from build123d import *

# Parameters (mm, degrees)
F0_W          = 20
F0_H          = 20
F1_DEPTH      = 20
F2_W          = 15.5
F2_H          = 15.5
F3_DEPTH      = 25
F3_DEPTH_BACK = 25
F4_W          = 2.25
F4_H          = 20
F5_DEPTH      = 15
F6_W          = 2.25
F6_H          = 35
F7_DEPTH      = 20
F8_R          = 3.25
F9_DEPTH      = 25
F9_DEPTH_BACK = 25
F10_R         = 1.75
F11_DEPTH     = 5
F12_R         = 10


with BuildPart() as f1:
    # F0 (on Top) → F1 (new body)
    with BuildSketch(Plane.XY):
        with Locations((10, 10)):
            Rectangle(F0_W, F0_H)
    extrude(amount=F1_DEPTH)

    # F2 (on face) → F3 (cut, two sides)
    with BuildSketch(Plane.XZ) as f3_sk:
        with Locations((10, 10)):
            Rectangle(F2_W, F2_H)
    extrude(amount=F3_DEPTH, mode=Mode.SUBTRACT)
    extrude(f3_sk.sketch, amount=-F3_DEPTH_BACK, mode=Mode.SUBTRACT)

    # F4 (on face) → F5 (join)
    with BuildSketch(Plane.XY.offset(20)):
        with Locations((1.125, 10)):
            Rectangle(F4_W, F4_H)
    extrude(amount=F5_DEPTH)

    # F6 (on face) → F7 (join)
    with BuildSketch(Plane(origin=(0, 20, 0), x_dir=(-1, 0, 0), z_dir=(0, 1, 0))):
        with Locations((-1.125, 17.5)):
            Rectangle(F6_W, F6_H)
    extrude(amount=F7_DEPTH)

    # F8 (on face) → F9 (cut, two sides)
    with BuildSketch(Plane.YZ.offset(2.25)) as f9_sk:
        with Locations((30, 22.25)):
            Circle(F8_R)
    extrude(amount=-F9_DEPTH, mode=Mode.SUBTRACT)
    extrude(f9_sk.sketch, amount=-F9_DEPTH_BACK, mode=Mode.SUBTRACT)

    # F10 (on face) → F11 (cut)
    with BuildSketch(Plane.YZ.offset(20)):
        with Locations((10, 10)):
            Circle(F10_R)
    extrude(amount=-F11_DEPTH, mode=Mode.SUBTRACT)

    # F12
    f12_edges = [f1.edges().sort_by_distance(p)[0] for p in [
        (1.125, 40, 35),
    ]]
    fillet(f12_edges, radius=F12_R)


solid = f1.part
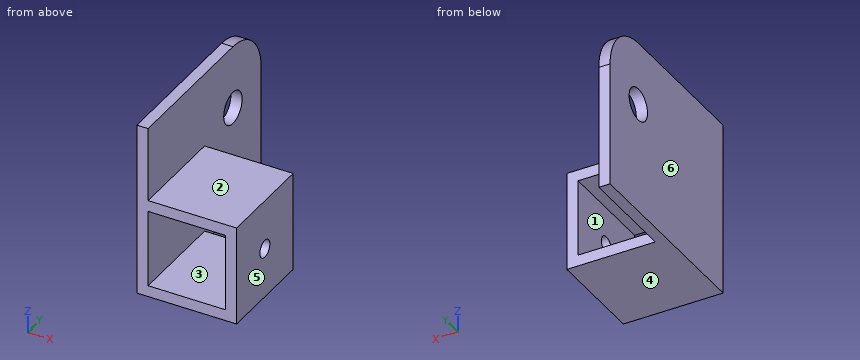
Can you work these out from the model? Positions are in its coordinate system, mm. Face numbers are marked on the shaded views. A direction names the side the tool comes from. Round coordinates to 2 decimals unless told otherwise and drop trailing zeros. Write each loop counter-clockwise with the first axis right and the second up, starting at its lowest first coordinate (ties: lowest second). Pieces come first, ordered by that corner, then holes. Notation, with made-up numbers: M 0.25,8.25 L 12.25,8.25 A33 cw 12.25,44.25 Z; hole C 64,-34.5 d9. An arc over 180 degrees is marked long. Use CSV: the item, a comma, the result in double quotes.
(1) I'm going to push flat-ended pins straight in: pin 1 (10.5 mm diameter, centred on y = 30, z = 22.25, fed in from -X); pin 2 (2 mm diameter, centred on x = 14, y = 21.5, fed in from +Z); pin 3 (1.5 mm diameter, centred on x = 15, y = 5.5, fed in from +Z); pin 4 (8 mm diameter, centred on y = 33.5, z = 17.5, fed in from +X). Where does each tip first touch, or does it pass through?
Check values:
pin 1,"x = 0"
pin 2,"through"
pin 3,"z = 20"
pin 4,"x = 2.25"
(2) Imagine slicing it at A-A (z = 22.25). Write out the boundary of the cut face in (x, y), plus the area to 3 significant figures.
Check values:
outline,"M 0,0 L 2.25,0 L 2.25,26.75 L 0,26.75 Z; M 0,33.25 L 2.25,33.25 L 2.25,40 L 0,40 Z"
area,"75.4 mm^2"
(3) Imagine slicing it at B-B (y = 4.5). Write out the boundary of the cut face in (x, z).
Check values:
outline,"M 0,0 L 20,0 L 20,20 L 2.25,20 L 2.25,35 L 0,35 Z; hole M 2.25,2.25 L 17.75,2.25 L 17.75,17.75 L 2.25,17.75 Z"
(4) We'd pull the mould along X, two halves only. Please class the marked faces 3, 4, 5 and 6: +X half, -X half, draft (parallel to the pull), parting line (faces both ways), or undercut.
Check values:
face 3,"undercut"
face 4,"draft"
face 5,"+X half"
face 6,"-X half"
(5) I need wall thicknesses on line 1 along X through (y, z) = (10.5, 5); line 2 along Z through (x, y) = (0.8, 30). Which ranges of each line are inside material? Lowest first, please.
Check values:
line 1,"0 to 2.25, 17.75 to 20"
line 2,"0 to 19, 25.5 to 35"
(6) Imagine slicing it at C-C (x = 17). Write out the boundary of the cut face in (y, z), plus the area to 3 significant figures.
Check values:
outline,"M 0,0 L 20,0 L 20,2.25 L 0,2.25 Z; M 0,17.75 L 20,17.75 L 20,20 L 0,20 Z"
area,"90.0 mm^2"
(7) On a 3-axis mill with a long thin cutter (end or side, diameter ignored), from which of +Z, -Z, +X, -X, +Y, -Y can I reach the whole of each face in a straight line? I mean the marked faces 1 and 2. Say none if no direction works.
Check values:
face 1,"+Y, -Y"
face 2,"+Z, +X, +Y, -Y"
(8) Imagine slicing it at D-D (z = 10). Write out the boundary of the cut face in (x, y), plus the area to 3 significant figures.
Check values:
outline,"M 0,0 L 2.25,0 L 2.25,40 L 0,40 Z; M 17.75,0 L 20,0 L 20,8.25 L 17.75,8.25 Z; M 17.75,11.75 L 20,11.75 L 20,20 L 17.75,20 Z"
area,"127 mm^2"
